Answer from the drawing. Dimensions are ordinates in mm from the lowest x, y and z of the part. A direction names the side the tool comes from. Round coordinates to 2 decimals unless told otherwise and drop trailing zeros. Loops run counter-clockwise (first coordinate to the right, second up) from the corner with the lowest first, then second, coordinate; pieces in that order, holes last. Notation, with made-up numbers: (81.25, -25.5) - (126.25, -25.5) arc R6 ccw to (126.25, -14.5) - close; hole circle Ø4 at (11.25, 83.5). An arc over 180 degrees is marked (long way). Return JSON: item names as keys, results as strings.
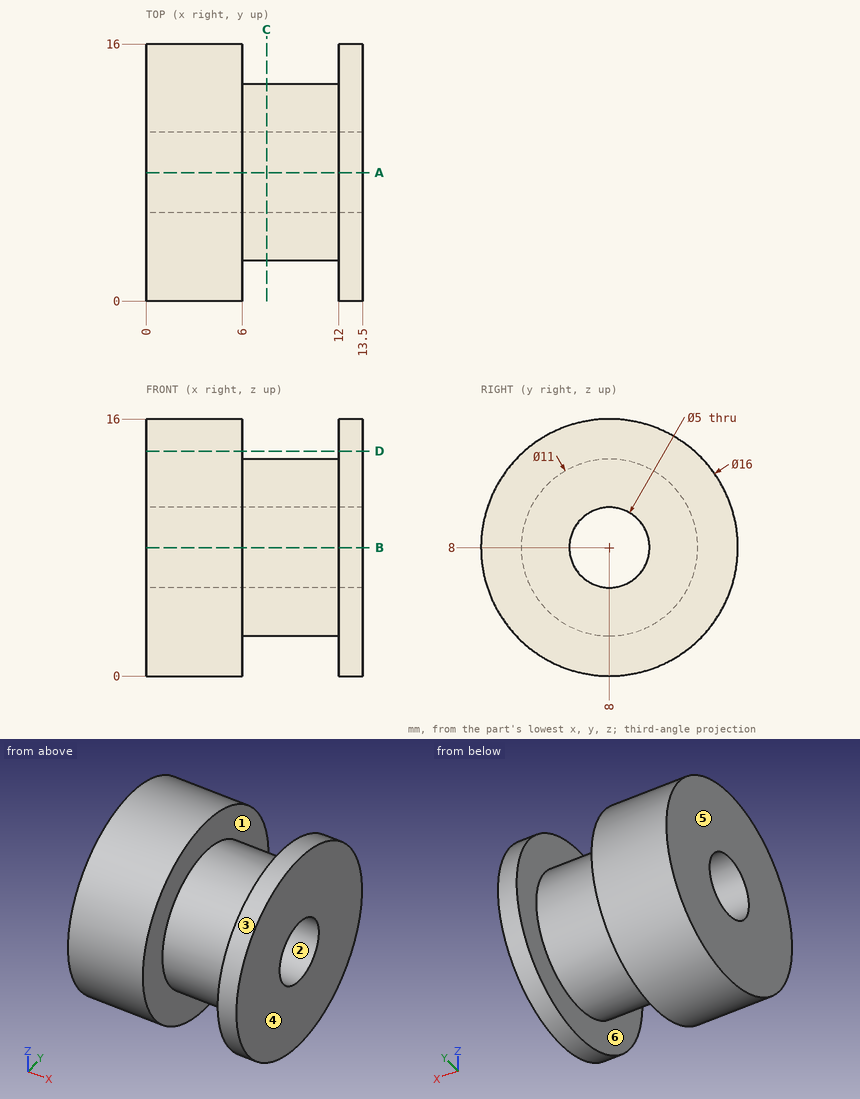
1) Flat-ended cylindrical pins translate along their axes: pin 1 (1.5 mm diameter, centred on x = 8.5, z = 2.5, fed in from -Y); pin 2 (6 mm diameter, centred on x = 8.5, z = 3, fed in from -Y); pin 3 (3 mm diameter, centred on x = 11.5, z = 4.5, fed in from +Y). Find the tip coordinate at first contact, or state that the pin passes through.
Verdict:
{"pin 1": "stops at y = 5.23", "pin 2": "stops at y = 0.73", "pin 3": "stops at y = 15.72"}
2) Find the intervals of material crossed by L1, parallel to Y at x = 4.5, z = 8; L2, parallel to Y at x = 8.25, z = 8; L3, parallel to X at y = 3.25, z = 13, in increasing order.
Verdict:
{"L1": "y = 0 to 5.5, 10.5 to 16", "L2": "y = 2.5 to 5.5, 10.5 to 13.5", "L3": "x = 0 to 6, 12 to 13.5"}
3) Determine the mould class of the marked faces 3, 4, 5 and 6 for opening direction X: pulls with the +X half, pulls with the -X half, needs draft (parallel to the pull), parting line crosses it, or undercut.
Verdict:
{"face 3": "needs draft", "face 4": "pulls with the +X half", "face 5": "pulls with the -X half", "face 6": "undercut"}
4) Section C-C (x = 7.5) is taken. Give the vertices of the cut face in (y, z), and give its area (3 significant figures).
Verdict:
{"outline": "circle Ø11 at (8, 8); hole circle Ø5 at (8, 8)", "area": "75.4 mm2"}
5) A tool of negligible diameter and unlimited length cuts with its end or side. For the marked faces 1 and 2, from which of +Z, -Z, +X, -X, +Y, -Y can it reach the whole face along a straight path? Write none if from no direction.
Verdict:
{"face 1": "none", "face 2": "+X, -X"}
6) Section A-A (y = 8) is taken. Give the vertices of the cut face in (x, z), and give its area (4 significant figures).
Verdict:
{"outline": "(0, 0) - (6, 0) - (6, 2.5) - (12, 2.5) - (12, 0) - (13.5, 0) - (13.5, 5.5) - (0, 5.5) - close; (0, 10.5) - (13.5, 10.5) - (13.5, 16) - (12, 16) - (12, 13.5) - (6, 13.5) - (6, 16) - (0, 16) - close", "area": "118.5 mm2"}
7) Section D-D (z = 14) is taken. Give the vertices of the cut face in (x, y), and give its area (3 significant figures).
Verdict:
{"outline": "(0, 2.71) - (6, 2.71) - (6, 13.29) - (0, 13.29) - close; (12, 2.71) - (13.5, 2.71) - (13.5, 13.29) - (12, 13.29) - close", "area": "79.4 mm2"}
